```python
from build123d import *

# Parameters (mm, degrees)
F0_R             = 25.4
F1_DEPTH         = 15.5575
F2_R             = 3.175
F3_DEPTH         = 31.116
F4_R             = 20.32
F5_DEPTH         = 8.89
F6_R             = 1.4224
F7_DEPTH         = 12.7
F9_R             = 4.7625
F9_R_2           = 3.175
F10_DEPTH        = 3.175
F10_COPIES_COUNT = 6
F11_R            = 3.175
F12_DEPTH        = 15.875
F12_COPIES_COUNT = 6


# Not quite as in the source:
# - a pattern or mirror of a feature is missing from the dataset's text; its kind, count and spacing are read off the source's solid


with BuildPart() as f1:
    # F0 (on Right) → F1 (new body, symmetric)
    with BuildSketch(Plane.YZ):
        Circle(F0_R)
    extrude(amount=F1_DEPTH, both=True)

    # F2 (on face) → F3 (cut, through all)
    with BuildSketch(Plane.YZ.offset(15.5575)):
        Circle(F2_R)
    extrude(amount=-F3_DEPTH, mode=Mode.SUBTRACT)

    # F4 (on face) → F5 (cut)
    with BuildSketch(Plane.YZ.offset(15.5575)):
        Circle(F4_R)
    extrude(amount=-F5_DEPTH, mode=Mode.SUBTRACT)

    # F6 (on face) → F7 (cut)
    with BuildSketch(Plane.YZ.offset(6.6675)):
        with Locations((14.6812, 0)):
            Circle(F6_R)
        with Locations((7.3406, -12.714292158)):
            Circle(F6_R)
        with Locations((-7.3406, -12.714292158)):
            Circle(F6_R)
        with Locations((-14.6812, 0)):
            Circle(F6_R)
        with Locations((-7.3406, 12.714292158)):
            Circle(F6_R)
        with Locations((7.3406, 12.714292158)):
            Circle(F6_R)
    extrude(amount=-F7_DEPTH, mode=Mode.SUBTRACT)

    # F9 (on offset) → F10 (cut)
    with BuildSketch(Plane.XY.offset(25.4)):
        Circle(F9_R)
        Circle(F9_R_2, mode=Mode.SUBTRACT)
        Circle(F9_R_2)
    f10 = extrude(amount=-F10_DEPTH, mode=Mode.SUBTRACT)

    # F10_copies: F10 ×6 about axis
    f10_copies_axis = Axis((0, 0, 0), (1, 0, 0))
    for i in range(1, F10_COPIES_COUNT):
        add(f10.rotate(f10_copies_axis, i * 360 / F10_COPIES_COUNT), mode=Mode.SUBTRACT)

    # F11 (on face) → F12 (cut)
    with BuildSketch(Plane.XY.offset(22.225)):
        Circle(F11_R)
    f12 = extrude(amount=-F12_DEPTH, mode=Mode.SUBTRACT)

    # F12_copies: F12 ×6 about axis
    f12_copies_axis = Axis((0, 0, 0), (1, 0, 0))
    for i in range(1, F12_COPIES_COUNT):
        add(f12.rotate(f12_copies_axis, i * 360 / F12_COPIES_COUNT), mode=Mode.SUBTRACT)


solid = f1.part
```
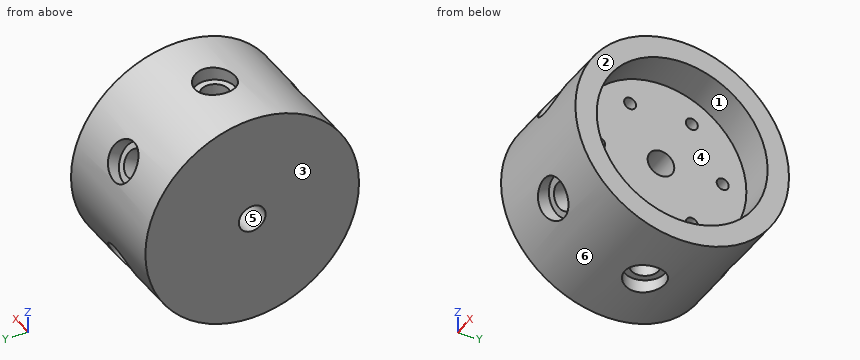
Verification items for the finished model (mm, model axes). Face numbers are marked on the shaded views. A direction names the side the tool comes from. Give positions to 0.01 mm unless a question says otherwise; leave off trailing zeros. Order: outer loops, then holes, each group sorted by start corner. A loop starts at its lowest first (then second) coordinate and runs counter-clockwise, first axis right, second up. Notation, with made-up numbers: (58, -2) -> (84, -2) arc R22 ccw to (84, 11) -> close; hole circle Ø5 at (-17.75, -15). An arc over 180 degrees is marked (long way). One line per item, written item: value.
(1) Draft check along Y on the marked faces 3, 4, 5 and 6. Enter one of: pulls with the +Y half, pulls with the -Y half, needs draft (parallel to the pull), parting line crosses it, or undercut.
Final values:
face 3: needs draft
face 4: undercut
face 5: undercut
face 6: parting line crosses it
(2) Scan lines: line 1 along X through (y, z) = (0, 24); line 2 along Z through (x, y) = (2, 6.5); line 3 along Z through (x, y) = (-1, -5). Record each from-to range of solid material in increasing order. Write a range as [from, to].
Final values:
line 1: [-15.56, -4.76], [4.76, 15.56]
line 2: [-24.55, -13.86], [-11.57, -6.6], [-1.44, 1.44], [6.6, 11.57], [13.86, 24.55]
line 3: [-24.9, -6.37], [-4.04, 4.04], [6.37, 24.9]
(3) Sectioned sample at C-C on y = -15. Count the separate pieces of the cut face and the enclosed holes in it, then the cut area to 3 significant figures.
Final values:
separate pieces: 1
enclosed holes: 2
area: 924 mm^2
(4) Tool access check on the marked faces 1 and 2. Record the directions out of +Z, -Z, +X, -X, +Y, -Y that give a thin tool (end or side, any length) a straight path to the whole face; none if there is none.
Final values:
face 1: +X
face 2: +Z, -Z, +X, +Y, -Y
(5) Gauge pin test, flat ends, axial feed: pin 1 (10 mm diameter, centred on y = 0, z = 0, fed in from +X); pin 2 (8.5 mm diameter, centred on x = 0, y = 0, fed in from +Z) (3 decimals); pin 3 (1.5 mm diameter, centred on x = 3, z = -9.5, fed in from +Y). Record the tip position at first contact, or that the pin passes through.
Final values:
pin 1: x = 6.67
pin 2: z = 22.225
pin 3: y = 23.85
(6) Sectioned sample at B-B on x = -7.5. Record the cut outline in (y, z) (3 decimals), then the cut area to 3 significant figures.
Final values:
outline: circle Ø50.8 at (0, 0); hole circle Ø6.35 at (0, 0)
area: 2,000 mm^2
